Autodesk Inventor part; units mm, degrees
ref_plane "YZ Plane" through (0, 0, 0) normal (1, 0, 0) x (0, 1, 0)
ref_plane "XZ Plane" through (0, 0, 0) normal (0, 1, 0) x (-1, 0, 0)
ref_plane "XY Plane" through (0, 0, 0) normal (0, 0, 1) x (1, 0, 0)
sketch "Sketch1" plane through (0, 0, 0) normal (0, 0, 1) x (1, 0, 0)
  line L0 (5.4993, 0) -> (2.7496, -4.7625)
  line L1 (2.7496, -4.7625) -> (-2.7496, -4.7625)
  line L2 (-2.7496, -4.7625) -> (-5.4993, 0)
  line L3 (-5.4993, 0) -> (-2.7496, 4.7625)
  line L4 (-2.7496, 4.7625) -> (2.7496, 4.7625)
  line L5 (2.7496, 4.7625) -> (5.4993, 0)
  circle A0 centre (0, 0) radius 0.0127
  dimension "d0" = 9.525
  dimension "d6" = 0.0254
extrude "Extrusion2" add sketch "Sketch1" along normal mid plane 88.9
sketch "Sketch4" plane through (0, 0, -44.45) normal (0, 0, -1) x (-1, 0, 0)
  circle A0 centre (0, 0) radius 0.0127
  circle A1 centre (0, 0) radius 12.7
  dimension "d10" = 25.4
extrude "Extrusion4" add sketch "Sketch4" against normal blind 19.05
thicken "Reduce Hex Shaft" operation add thickness 0.127 both sides no extend neighbours yes toward (0, -1, 0) faces at (0.9165, 4.7625, -2.1167) (4.5827, 1.5875, -2.1167) (3.6662, -3.175, -2.1167) (-3.6662, 3.175, -2.1167) (-4.5827, -1.5875, -2.1167) (-0.9165, -4.7625, -2.1167)
sketch "Sketch5" plane through (0, 0, -25.4) normal (0, 0, 1) x (1, 0, 0)
  circle A0 centre (0, 0) radius 6.35
  dimension "d15" = 12.7
extrude "Extrusion5" add sketch "Sketch5" along normal blind 6.35
thicken "Reduce Base Bushing" operation add thickness 0.127 both sides no extend neighbours yes toward (-0.9967573, 0.0804666, 0) faces at (6.3294, -0.511, -21.1667)
equation "\"d0\" = hexSize"
equation "\"d4\" = length"
equation "\"d13\" = printOffset"
equation "\"d14\" = printOffset"
equation "\"d15\" = bushingForBaseHole"
equation "\"d16\" = sideOfBase"
equation "\"d20\" = printOffset"
equation "\"d21\" = printOffset"
equation "\"hexSize\" = 9.525"
equation "\"length\" = 88.9"
equation "\"printOffset\" = 0.127"
equation "\"bushingForBaseHole\" = 12.7"
equation "\"sideOfBase\" = 6.35"
properties part number "3_8x3-inchHexShaft"
The model under review builds one solid part; all positions refer to its coordinate system, in mm. A direction names the side the tool comes from. Round coordinates to 2 decimals unless told otherwise and drop trailing zeros. Loops run counter-clockwise (first coordinate to the right, second up) from the corner with the lowest first, then second, coordinate; pieces in that order, holes last. Notation, with made-up numbers: (50, 2.5) - (82, 2.5) arc R34 cw to (82, 38.5) - close; hole circle Ø4 at (26, 62.5). An arc over 180 degrees is marked (long way). Write each question's results on one line, items separated by ' | '. Start each with the question number.
Q1. Insertion check: P1, Ø4, axis at x = -1.5, z = 21, coming from the -Y side; P2, Ø4.5, axis at x = -1, z = 25.5, coming from the +Y side; P3, Ø6, axis at x = 7.5, z = -1, coming from the +Y side. Each pin has a flat end and moves straight along its axis. Give the tip position at first contact, or say it passes through.
Q2. Take a section at C-C on x = -4.5. Give the boundary of the cut face in (y, z), plus the area to 3 significant figures.
Q3. Wall thickness on line 1 along Z through (x, y) = (-0.25, 8.75); line 2 along Y through (x, z) = (-2, 8.5); line 3 along Z through (x, y) = (4.5, -2.25): over which ranges is each line inside the solid? List them lowest first. Write a range as [from, to].
Q4. Tool access review of faces 1 (the flat face through (4.03, -2.29, 12.26)), 2 (the flat face through (-3, 6, -25.4)), 3 (the flat face through (-3.996, -2.35, 12.256)): name each direction out of +Z, -Z, +X, -X, +Y, -Y from which nothing blocks a thin tool from reaching the whole face with its end or side.
Q5. Take a section at D-D on y = 8.5. Give the boundary of the cut face in (x, z), plus the area to 3 significant figures.
Q6. Take a section at B-B on y = 3.5. Give the boundary of the cut face in (x, z).
Data:
1) P1: stops at y = -4.64 | P2: stops at y = 4.64 | P3: stops at y = 1.48
2) outline: (-11.88, -44.45) - (11.88, -44.45) - (11.88, -25.4) - (4.3, -25.4) - (4.3, -19.05) - (1.48, -19.05) - (1.48, 44.45) - (-1.48, 44.45) - (-1.48, -19.05) - (-4.3, -19.05) - (-4.3, -25.4) - (-11.88, -25.4) - close | area: 695 mm²
3) line 1: z = [-44.45, -25.4] | line 2: y = [-4.64, 4.64] | line 3: z = [-44.45, -19.05]
4) face 1: +Z, +X, -Y | face 2: +Z | face 3: +Z, -X, -Y
5) outline: (-9.44, -44.45) - (9.44, -44.45) - (9.44, -25.4) - (-9.44, -25.4) - close | area: 360 mm²
6) outline: (-12.21, -44.45) - (12.21, -44.45) - (12.21, -25.4) - (5.15, -25.4) - (5.15, -19.05) - (3.33, -19.05) - (3.33, 44.45) - (-3.33, 44.45) - (-3.33, -19.05) - (-5.15, -19.05) - (-5.15, -25.4) - (-12.21, -25.4) - close
